Model file for the job. Use its own axes, mm. Face numbers are marked on the shaded views. A direction names the side the tool comes from. Give positions to 0.01 mm unless a question says otherwise; leave off trailing zeros. One line per item, written item: value. Start each with the question number.
(1) Drop a flat-ended pin along its axis: P1, Ø3, axis at x = 0.5, y = -0.5, coming from the -Z side. Give the stop position or say it passes through.
(2) 3-axis set-ups, long thin cutter, end or side, ignore diameter. For the marked faces 1 and 2: which of +Z, -Z, +X, -X, +Y, -Y reach the whole face in a straight line?
(3) Probe L1, parallel to Z at x = 0.25, y = 3; L2, parallel to X at y = 1, z = 0.2; L3, parallel to Y at x = -2.5, z = 0.05. List the from-to ranges inside material, lowest first.
(4) Mould opens along Y. For the marked faces 3, 4 and 5 say: pulls with the +Y half, pulls with the -Y half, needs draft (parallel to the pull), parting line crosses it, or undercut.
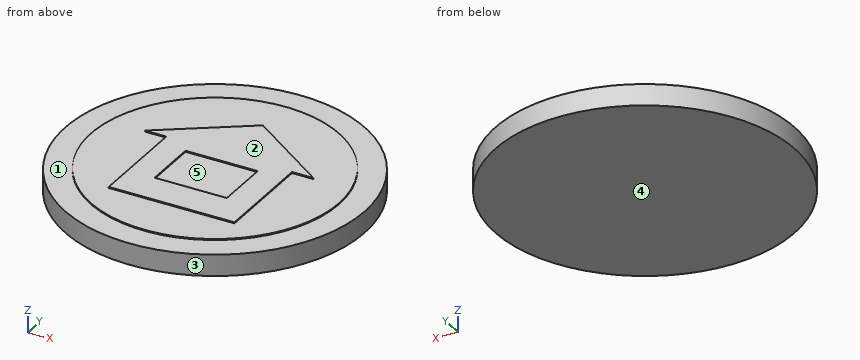
from build123d import *

# Parameters (mm, degrees)
F0_R     = 3.550157
F1_DEPTH = 0.508
F2_R     = 2.943
F3_DEPTH = 0.0254
F4_W     = 1.713301
F4_H     = 1.288881
F5_DEPTH = 0.0254


with BuildPart() as f1:
    # F0 (on Top) → F1 (new body)
    with BuildSketch(Plane.XY):
        Circle(F0_R)
    extrude(amount=F1_DEPTH)

    # F2 (on face) → F3 (join)
    with BuildSketch(Plane.XY.offset(0.508)):
        Circle(F2_R)
    extrude(amount=F3_DEPTH)

    # F4 (on face) → F5 (join)
    with BuildSketch(Plane.XY.offset(0.5334)):
        Polygon((-1.502313, -1.794855), (1.480988, -1.794855), (1.480988, 0.612127), (1.989505, 0.612127), (0, 2.002074), (-2.010831, 0.612127), (-1.502313, 0.612127), align=None)
        with Locations((-0.010663, -0.349021)):
            Rectangle(F4_W, F4_H, mode=Mode.SUBTRACT)
    extrude(amount=F5_DEPTH)


solid = f1.part
Answers follow:
1. P1: stops at z = 0
2. face 1: +Z
2. face 2: +Z, +X, -X, +Y, -Y
3. L1: z = 0 to 0.51
3. L2: x = -3.41 to 3.41
3. L3: y = -2.52 to 2.52
4. face 3: parting line crosses it
4. face 4: needs draft
4. face 5: undercut
